Read the model definition and answer for the solid it produces. Units are mm, in the model's axes. Face numbers are marked on the shaded views. A direction names the side the tool comes from. Give positions to 0.01 mm unless a question says otherwise; leave off trailing zeros. Order: outer loops, then holes, each group sorted by start corner. A loop starts at its lowest first (then second) coordinate and runs counter-clockwise, first axis right, second up. Notation, with made-up numbers: (-34, 86) - (-25, 86) arc R19 cw to (-25, 90) - close; hole circle Ø7 at (88, 20). An arc over 180 degrees is marked (long way). Write item = value, one per line.
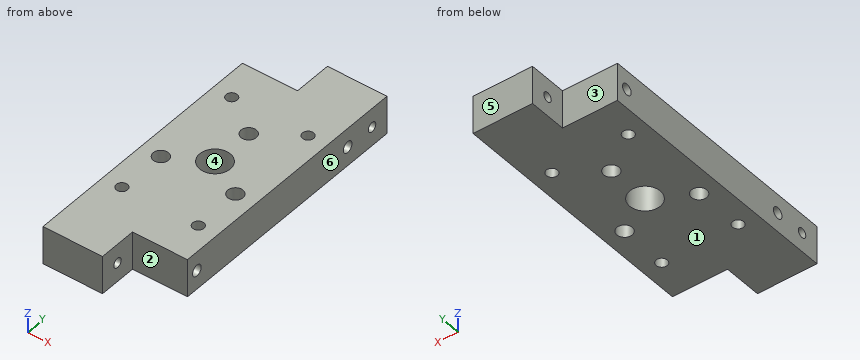
Autodesk Inventor part; units mm, degrees
ref_plane "YZ Plane" through (0, 0, 0) normal (1, 0, 0) x (0, 1, 0)
ref_plane "XZ Plane" through (0, 0, 0) normal (0, 1, 0) x (-1, 0, 0)
ref_plane "XY Plane" through (0, 0, 0) normal (0, 0, 1) x (1, 0, 0)
sketch "Sketch1" plane through (0, 0, 0) normal (0, 0, 1) x (1, 0, 0)
  line L0 (-19.05, -48.7045) -> (19.05, -48.7045)
  line L1 (19.05, -48.7045) -> (19.05, 48.7045)
  line L2 (19.05, 48.7045) -> (-19.05, 48.7045)
  line L3 (-19.05, 48.7045) -> (-19.05, -48.7045)
  line L4 (-19.05, -48.7045) -> (19.05, 48.7045) construction
  line L5 (19.05, -48.7045) -> (-19.05, 48.7045) construction
  point P0 (0, 0)
  dimension "d0" = 38.1
  dimension "d1" = 97.409
extrude "Extrusion1" add sketch "Sketch1" along normal blind 12.7
sketch "Sketch2" plane through (0, 0, 12.7) normal (0, 0, 1) x (1, 0, 0)
  line L0 (-19.05, 48.7045) -> (-0.762, 48.7045)
  line L1 (-0.762, 48.7045) -> (-0.762, 36.0045)
  line L2 (-0.762, 36.0045) -> (-19.05, 36.0045)
  line L3 (-19.05, 36.0045) -> (-19.05, 48.7045)
  point P0 (0, 0)
  dimension "d4" = 18.288
  dimension "d5" = 12.7
extrude "Extrusion2" cut sketch "Sketch2" against normal blind 12.7
sketch "Sketch3" plane through (0, 0, 12.7) normal (0, 0, 1) x (1, 0, 0)
  line L0 (19.05, -48.7045) -> (0.762, -48.7045)
  line L1 (0.762, -48.7045) -> (0.762, -36.0045)
  line L2 (0.762, -36.0045) -> (19.05, -36.0045)
  line L3 (19.05, -36.0045) -> (19.05, -48.7045)
  point P0 (0, 0)
  dimension "d8" = 18.288
  dimension "d9" = 12.7
extrude "Extrusion3" cut sketch "Sketch3" against normal blind 12.7
sketch "Sketch4" plane through (0, 0, 12.7) normal (0, 0, 1) x (1, 0, 0)
  circle A0 centre (0, 0) radius 5.08
  dimension "d12" = 10.16
extrude "Extrusion4" cut sketch "Sketch4" against normal blind 12.7
sketch "Sketch5" plane through (19.05, 48.7045, 12.7) normal (1, 0, 0) x (0, 0, -1)
  line L0 (12.7, -97.409) -> (12.7, 0)
  line L1 (12.7, 0) -> (0, 0)
  line L2 (0, -84.709) -> (0, 0)
  line L3 (0, -12.7) -> (12.7, -12.7)
  circle A0 centre (6.35, -6.35) radius 1.5875
  point P0 (12.7, -48.7045)
  dimension "d16" = 3.175
  dimension "d17" = 6.35
  dimension "d18" = 6.35
  dimension "d19" = 6.35
  dimension "d20" = 6.35
extrude "Extrusion5" cut sketch "Sketch5" against normal blind 34.29 contours A0
sketch "Sketch9" plane through (-19.05, -48.7045, 0) normal (-1, 0, 0) x (0, 0, 1)
  line L0 (0, 0) -> (12.7, 0)
  line L1 (12.7, 84.709) -> (12.7, 0)
  line L2 (12.7, 12.709) -> (0, 12.709)
  circle A0 centre (6.35, 6.35) radius 1.5875
  line L3 (12.7, 12.7) -> (0, 12.7)
  point P0 (0, 48.7045)
  dimension "d34" = 3.175
  dimension "d35" = 6.35
  dimension "d40" = 6.35
  dimension "d41" = 6.35
extrude "Extrusion9" cut sketch "Sketch9" against normal blind 20.701
sketch "Sketch10" plane through (0, 0, 12.7) normal (0, 0, 1) x (1, 0, 0)
  circle A0 centre (0, 0) radius 5.08
  line L0 (0.762, -36.0045) -> (19.05, -36.0045)
  line L1 (4.0695, 16.6582) -> (16.4611, -4.8048)
  line L2 (12.3917, -11.8533) -> (-12.3917, -11.8533)
  line L3 (-16.4611, -4.8048) -> (-4.0695, 16.6582)
  line L4 (-1.524, 36.0045) -> (-1.524, -36.0045) construction
  arc A1 (-16.4611, -4.8048) -> (-12.3917, -11.8533) centre (-12.3917, -7.1543) ccw
  arc A2 (4.0695, 16.6582) -> (-4.0695, 16.6582) centre (0, 14.3087) ccw
  arc A3 (12.3917, -11.8533) -> (16.4611, -4.8048) centre (12.3917, -7.1543) ccw
  circle A4 centre (-12.3917, -7.1543) radius 2.54
  circle A5 centre (0, 14.3087) radius 2.54
  circle A6 centre (12.3917, -7.1543) radius 2.54
  point P0 (-0.762, 36.0045)
  point P1 (0, 23.7067)
  point P2 (20.5306, -11.8533)
  point P3 (-20.5306, -11.8533)
  dimension "d52" = 35.56
  dimension "d53" = 4.699
  dimension "d54" = 4.699
  dimension "d55" = 5.08
  dimension "d56" = 5.08
  dimension "d57" = 5.08
extrude "Extrusion11" cut sketch "Sketch10" against normal blind 12.7 contours A4 | A5 | A6
sketch "Sketch11" plane through (19.05, 48.7045, 12.7) normal (1, 0, 0) x (0, 0, -1)
  circle A0 centre (6.35, -16.7) radius 1.85
  circle A1 centre (6.35, -80.7) radius 1.85
  point P0 (12.7, -48.7045)
extrude "Extrusion12" cut sketch "Sketch11" against normal blind 38.1
sketch "Sketch12" plane through (0, 0, 12.7) normal (0, 0, 1) x (1, 0, 0)
  line L0 (0.762, -36.0045) -> (19.05, -36.0045)
  line L1 (19.05, -36.0045) -> (19.05, 48.7045)
  line L2 (-0.762, 36.0045) -> (-19.05, 36.0045)
  line L3 (-19.05, 36.0045) -> (-19.05, -48.7045)
  circle A0 centre (-12.7, 23.3045) radius 1.8542
  circle A1 centre (12.7, 23.3045) radius 1.8542
  circle A2 centre (12.7, -23.3045) radius 1.8542
  circle A3 centre (-12.7, -23.3045) radius 1.8542
  dimension "d62" = 3.7084
  dimension "d64" = 6.35
  dimension "d65" = 12.7
  dimension "d66" = 3.7084
  dimension "d67" = 12.7
  dimension "d68" = 6.35
  dimension "d69" = 3.7084
  dimension "d70" = 6.35
  dimension "d71" = 12.7
  dimension "d72" = 3.7084
  dimension "d73" = 6.35
  dimension "d74" = 12.7
extrude "Extrusion13" cut sketch "Sketch12" against normal blind 12.7
equation "\"d17\" = d18"
equation "\"d19\" = d20"
equation "\"d40\" = d41"
properties part number "MotorMount"
1. For the marked faces 1, 2 and 3, determine the directions among +Z, -Z, +X, -X, +Y, -Y from which every point of the face is accessible in a straight line to the end or side of a thin tool.
Recorded:
face_1 = -Z, +X, -X, +Y, -Y
face_2 = +Z, -Z, +X, -Y
face_3 = +Z, -Z, -X, +Y
2. Section B-B (y = 0) is taken. Determine the outline of the cut face in (x, z).
Recorded:
outline = (-19.05, 0) - (-5.08, 0) - (-5.08, 12.7) - (-19.05, 12.7) - close; (5.08, 0) - (19.05, 0) - (19.05, 12.7) - (5.08, 12.7) - close
3. Section A-A (x = 12.7) is taken. Count the separate pieces of the cut face and the enclosed holes in it, and give its area (3 significant figures).
Recorded:
separate_pieces = 4
enclosed_holes = 3
area = 888 mm^2
4. Determine the mould class of the marked faces 4, 5 and 6 for opening direction Y: +Y half, -Y half, draft (parallel to the pull), parting line (faces both ways), or undercut.
Recorded:
face_4 = undercut
face_5 = +Y half
face_6 = draft
5. Straight lines are drawn through the part: L1, parallel to Y at x = 0, z = 0.75; L2, parallel to Y at x = -3.75, z = 6.35; L3, parallel to Z at x = -6, y = 32.5. For each, find the intervals that lie inside material, in ascending order. Write a range as [from, to].
Recorded:
L1 = [-48.7, -5.08], [5.08, 11.77], [16.85, 48.7]
L2 = [-48.7, -43.94], [-40.77, -33.85], [-30.15, -3.43], [3.43, 30.15], [33.85, 36]
L3 = [0, 4.57], [8.13, 12.7]
6. Flat-ended cylindrical pins translate along their axes: pin 1 (6.5 mm diameter, centred on x = 12.39, y = -7.15, fed in from -Z); pin 2 (6.5 mm diameter, centred on x = -11.5, z = 6.5, fed in from +Y); pin 3 (6.5 mm diameter, centred on y = 41.5, z = 7, fed in from -X). Find the tip coordinate at first contact, or state that the pin passes through.
Recorded:
pin_1 = 0
pin_2 = 36
pin_3 = -0.76
